```python
from build123d import *

# Parameters (mm, degrees)
F1_DEPTH = 5


with BuildPart() as f1:
    # F0 (on Front) → F1 (new body)
    with BuildSketch(Plane.XZ):
        with BuildLine():
            Line((23.776413, 7.725425), (28.531695, 9.27051))
            ThreePointArc((28.531695, 9.27051), (28.327614, 9.876553), (28.11066, 10.478109))
            Line((28.11066, 10.478109), (14.694631, 20.225425))
            Line((14.694631, 20.225425), (17.633558, 24.27051))
            ThreePointArc((17.633558, 24.27051), (17.112228, 24.640853), (16.583124, 25))
            Line((16.583124, 25), (0, 25))
            Line((0, 25), (0, 30))
            ThreePointArc((0, 30), (-0.639446, 29.993184), (-1.278602, 29.972741))
            Line((-1.278602, 29.972741), (-14.694631, 20.225425))
            Line((-14.694631, 20.225425), (-17.633558, 24.27051))
            ThreePointArc((-17.633558, 24.27051), (-18.146874, 23.889139), (-18.651946, 23.496913))
            Line((-18.651946, 23.496913), (-23.776413, 7.725425))
            Line((-23.776413, 7.725425), (-28.531695, 9.27051))
            ThreePointArc((-28.531695, 9.27051), (-28.722813, 8.660254), (-28.90088, 8.046063))
            Line((-28.90088, 8.046063), (-23.776413, -7.725425))
            Line((-23.776413, -7.725425), (-28.531695, -9.27051))
            ThreePointArc((-28.531695, -9.27051), (-28.327614, -9.876553), (-28.11066, -10.478109))
            Line((-28.11066, -10.478109), (-14.694631, -20.225425))
            Line((-14.694631, -20.225425), (-17.633558, -24.27051))
            ThreePointArc((-17.633558, -24.27051), (-17.112228, -24.640853), (-16.583124, -25))
            Line((-16.583124, -25), (0, -25))
            Line((0, -25), (0, -30))
            ThreePointArc((0, -30), (0.639446, -29.993184), (1.278602, -29.972741))
            Line((1.278602, -29.972741), (14.694631, -20.225425))
            Line((14.694631, -20.225425), (17.633558, -24.27051))
            ThreePointArc((17.633558, -24.27051), (18.146874, -23.889139), (18.651946, -23.496913))
            Line((18.651946, -23.496913), (23.776413, -7.725425))
            Line((23.776413, -7.725425), (28.531695, -9.27051))
            ThreePointArc((28.531695, -9.27051), (28.722813, -8.660254), (28.90088, -8.046063))
            Line((28.90088, -8.046063), (23.776413, 7.725425))
        make_face()
    extrude(amount=F1_DEPTH)


solid = f1.part
```
Build history of the part. All positions in model axes, mm. A direction names the side the tool comes from. Give positions to 0.01 mm unless a question says otherwise; leave off trailing zeros. Loops run counter-clockwise (first coordinate to the right, second up) from the corner with the lowest first, then second, coordinate; pieces in that order, holes last. Notation, with made-up numbers: (45.5, 86.5) -> (61.5, 86.5) arc R20 ccw to (61.5, 114.5) -> close; hole circle Ø5 at (4, 25). An arc over 180 degrees is marked (long way). One line per question, with ' | ' between items.
Q1. Cut at D-D, the plane z = 14. Write the cut outline in (x, y).
Filled sheet:
outline: (-21.74, -5) -> (23.26, -5) -> (23.26, 0) -> (-21.74, 0) -> close
Q2. Cut at C-C, the plane x = 10. Write the cut outline in (y, z), plus the area to 3 significant figures.
Filled sheet:
outline: (-5, -23.64) -> (0, -23.64) -> (0, 25) -> (-5, 25) -> close | area: 243 mm²
Q3. Drop flat-ended pins along their axis: pin 1 (2 mm diameter, centred on y = -2.5, z = 19, fed in from +X); pin 2 (1.5 mm diameter, centred on y = -3.5, z = 28.5, fed in from +X). Give the stop position or say it passes through.
Filled sheet:
pin 1: stops at x = 17.76 | pin 2: stops at x = 0
Q4. Pull direction Z, two halves, no side cores. Call faces 5 (the flat face through (-16.144, -2.465, 22.22)), 6 (the flat face through (-21.5, -2.46, -15.28)), 7 (the flat face through (16.144, -2.465, -22.22)): pulls with the +Z half, pulls with the -Z half, needs draft (parallel to the pull), parting line crosses it, or undercut.
Filled sheet:
face 5: pulls with the +Z half | face 6: undercut | face 7: pulls with the -Z half
Q5. Cut at A-A, the plane z = 22. Write the cut outline in (x, y), plus the area to 3 significant figures.
Filled sheet:
outline: (-19.14, -5) -> (-15.98, -5) -> (-15.98, 0) -> (-19.14, 0) -> close; (-12.25, -5) -> (15.98, -5) -> (15.98, 0) -> (-12.25, 0) -> close | area: 157 mm²
Q6. Drill centre lines: line 1 along Z through (x, y) = (-16.5, -4.5); line 2 along X through (y, z) = (-3.7, 24); line 3 along Z through (x, y) = (-6.5, -4.25). Where is each one in solid material? Low to high. Write a range as [from, to].
Filled sheet:
line 1: z = [-25, -22.71], [-18.91, 22.71] | line 2: x = [-18, -17.44], [-9.5, 17.44] | line 3: z = [-25, 26.18]
Q7. Tool access for faces 1 (the flat face through (0, -2, -27)), 2 (the flat face through (26.121, -2.465, -8.487)), 3 (the flat face through (-26.121, -2.465, 8.487)), 4 (the flat face through (26.121, -2.465, 8.487)): list every direction of +Z, -Z, +X, -X, +Y, -Y with a clear straight run to the whole face (end or side of a thin tool).
Filled sheet:
face 1: -Z, -X, +Y, -Y | face 2: -Z, +Y, -Y | face 3: +Z, +Y, -Y | face 4: +X, +Y, -Y
